```python
from build123d import *

# Parameters (mm, degrees)
F0_W     = 110
F0_H     = 40
F0_W_2   = 107.6
F0_H_2   = 37.6
F1_DEPTH = 91.5
F2_DEPTH = 1.2
F3_R     = 2
F4_R     = 1


with BuildPart() as f1:
    # F0 (on Top) → F1 (new body)
    with BuildSketch(Plane.XY):
        with Locations((-18.294387, -26.759323)):
            Rectangle(F0_W, F0_H)
        with Locations((-18.294387, -26.759323)):
            Rectangle(F0_W_2, F0_H_2, mode=Mode.SUBTRACT)
    extrude(amount=F1_DEPTH)

    # F0 (on Top) → F2 (join)
    with BuildSketch(Plane.XY):
        with Locations((-18.294387, -26.759323)):
            Rectangle(F0_W, F0_H)
        with Locations((-18.294387, -26.759323)):
            Rectangle(F0_W_2, F0_H_2, mode=Mode.SUBTRACT)
        with Locations((-18.294387, -26.759323)):
            Rectangle(F0_W_2, F0_H_2)
    extrude(amount=F2_DEPTH)

    # F3
    f3_edges = [f1.edges().sort_by_distance(p)[0] for p in [
        (-73.294387, -46.759323, 45.75),
        (36.705613, -46.759323, 45.75),
        (36.705613, -6.759323, 45.75),
        (-73.294387, -6.759323, 45.75),
        (35.505613, -7.959323, 46.35),
        (-72.094387, -7.959323, 46.35),
        (-72.094387, -45.559323, 46.35),
        (35.505613, -45.559323, 46.35),
    ]]
    fillet(f3_edges, radius=F3_R)

    # F4
    f4_edges = [f1.edges().sort_by_distance(p)[0] for p in [
        (-72.094387, -26.759323, 1.2),
    ]]
    fillet(f4_edges, radius=F4_R)


solid = f1.part
```
The model under review builds one solid part; all positions refer to its coordinate system, in mm. A direction names the side the tool comes from. Give positions to 0.01 mm unless a question says otherwise; leave off trailing zeros. Loops run counter-clockwise (first coordinate to the right, second up) from the corner with the lowest first, then second, coordinate; pieces in that order, holes last. Notation, with made-up numbers: (31, 50.5) - (52, 50.5) arc R23 ccw to (52, 85.5) - close; hole circle Ø3 at (20.25, -9.75). An arc over 180 degrees is marked (long way). Answer as a JSON object with one key per item and string values.
Q1. Add section A-A on z = 29.5. State the section outline as (x, y) points.
Worked out:
{"outline": "(-73.29, -44.76) arc R2 ccw to (-71.29, -46.76) - (34.71, -46.76) arc R2 ccw to (36.71, -44.76) - (36.71, -8.76) arc R2 ccw to (34.71, -6.76) - (-71.29, -6.76) arc R2 ccw to (-73.29, -8.76) - close; hole (-72.09, -43.56) arc R2 ccw to (-70.09, -45.56) - (33.51, -45.56) arc R2 ccw to (35.51, -43.56) - (35.51, -9.96) arc R2 ccw to (33.51, -7.96) - (-70.09, -7.96) arc R2 ccw to (-72.09, -9.96) - close"}
Q2. For faces 1 (the flat face through (-72.094, -27, 46)), 2 (the flat face through (36.706, -27, 45)), list the 3-axis set-ups (+Z, -Z, +X, -X, +Y, -Y) from which the entire face can be reached by the end or side of a thin tool; tool diameter is ignored.
Worked out:
{"face 1": "+Z", "face 2": "+Z, -Z, +X, +Y, -Y"}
Q3. Mouldability with a two-part tool opening along Y and no side actions: class faces 3 (the flat face through (-19, -6.759, 45)), 4 (the flat face through (35.506, -27, 46)), 5 (the flat face through (-19, -7.959, 46)), 6 (the flat face through (-19, -7, 91.5)) as +Y half, -Y half, draft (parallel to the pull), parting line (faces both ways), or undercut.
Worked out:
{"face 3": "+Y half", "face 4": "undercut", "face 5": "undercut", "face 6": "draft"}
Q4. To check wall thickness, follow line 1 along Y through (x, z) = (17, 39); line 2 along X through (y, z) = (-13, 55); line 3 along Z through (x, y) = (16, -31). State the ranges of each line that lie inside material, in increasing order.
Worked out:
{"line 1": "y = -46.76 to -45.56, -7.96 to -6.76", "line 2": "x = -73.29 to -72.09, 35.51 to 36.71", "line 3": "z = 0 to 1.2"}
Q5. Add section B-B on y = -20. State the section outline as (x, z) points.
Worked out:
{"outline": "(-73.29, 0) - (36.71, 0) - (36.71, 91.5) - (35.51, 91.5) - (35.51, 2.2) arc R1 cw to (34.51, 1.2) - (-71.09, 1.2) arc R1 cw to (-72.09, 2.2) - (-72.09, 91.5) - (-73.29, 91.5) - close"}
Q6. Add section C-C on x = -56. State the section outline as (y, z) points, plus the area to 3 significant figures.
Worked out:
{"outline": "(-46.76, 0) - (-6.76, 0) - (-6.76, 91.5) - (-7.96, 91.5) - (-7.96, 2.2) arc R1 cw to (-8.96, 1.2) - (-44.56, 1.2) arc R1 cw to (-45.56, 2.2) - (-45.56, 91.5) - (-46.76, 91.5) - close", "area": "265 mm^2"}
